Input: part model. Units: mm. Frame: model coordinates. A direction names the side the tool comes from. Coordinates: 2 decimals unless noted, no trailing zeros. Write each loop counter-clockwise with the first axis right and the second up, starting at its lowest first coordinate (ties: lowest second). Pieces come first, ordered by that corner, then holes. Notation, with made-up numbers: M 43,53 L 92,53 A23 cw 92,70 Z; hole C 21,-35.75 d1. An arc over 180 degrees is marked long. Write each question's results on one line, items separated by ' | '. Start each with the question number.
1. Section query B-B, the plane y = 27.5. Output: boundary loops of the cut face in (x, z), and give its area (3 significant figures).
2. Ray query, probe 1 along Z at (x, y) = (49, 41.5); probe 2 along Z at (x, y) = (61, 1); probe 3 along X at (y, z) = (34.5, 34.5). Return the intervals inside material, ascending.
3. Set-up query: faces 1 (the flat face through (66, 1, 21)), 2 (the flat face through (4, 2, 21)), 3 (the cylindrical face through (54.57, 0.6, 21.29)). Return all of +Z, -Z, +X, -X, +Y, -Y with unobstructed straight access to the full face (end or side cutting, diameter ignored); none if empty.
4. Section query C-C, the plane z = 21. Output: boundary loops of the cut face in (x, y), and give its area (3 significant figures).
5. First-contact query: pin 1 (6 mm diameter, centred on y = 21, z = 11.5, fed in from +X); pin 2 (4 mm diameter, centred on x = 5.5, z = 21, fed in from +Y); pin 3 (18 mm diameter, centred on y = 16.5, z = 23.5, fed in from -X). Flat tips, straight axial feed; report the tip coordinate or a pass-through.
6. Pull-direction query (X, two-part tool) for faces 4 (the flat face through (10, 22, 21)), 5 (the cylindrical face through (62.45, 0.99, 35.94)), 6 (the cylindrical face through (56.6, 2.57, 21.29)); classes: +X half, -X half, draft (parallel to the pull), parting line (faces both ways), or undercut.
7. Section query D-D, the plane x = 5. Output: boundary loops of the cut face in (y, z).
8. Section query A-A, the plane x = 33. Output: boundary loops of the cut face in (y, z).
```python
from build123d import *

# Parameters (mm, degrees)
BOSS_EXTRU_1_DEPTH      = 42
D_GAGEMENT_M2_51_D      = 2.9
D_GAGEMENT_M21_D        = 2.4
ENL_V_MAT_EXTRU_1_REACH = 90.792
ESQUISSE6_R             = 11
CONG_1_R                = 2


with BuildPart() as part:
    # Esquisse1 → Boss.-Extru.1 (new body)
    with BuildSketch(Plane.XY):
        Polygon((0, 0), (12, 0), (12, 40), (54, 40), (54, 0), (66, 0), (66, 2), (56, 2), (56, 42), (10, 42), (10, 2), (0, 2), align=None)
    extrude(amount=BOSS_EXTRU_1_DEPTH)

    # Dégagement M2.51 (through all)
    with Locations(Plane(origin=(0, 2, 0), x_dir=(1, 0, 0), z_dir=(0, 1, 0))):
        with Locations((5, -6), (5, -36), (61, -6), (61, -36)):
            Hole(D_GAGEMENT_M2_51_D / 2)

    # Dégagement M21 (through all)
    with Locations(Plane(origin=(0, 42, 0), x_dir=(1, 0, 0), z_dir=(0, 1, 0))):
        with Locations((17, -5), (49, -37), (17, -37), (49, -5)):
            Hole(D_GAGEMENT_M21_D / 2)

    # Esquisse6 → Enlèv. mat.-Extru.1 (cut, up to next)
    with BuildSketch(Plane(origin=(0, 42, 0), x_dir=(1, 0, 0), z_dir=(0, 1, 0)), mode=Mode.PRIVATE) as enl_v_mat_extru_1_sk1:
        with Locations(Location((33, -21, 0), (0, 0, 270))):
            Circle(ESQUISSE6_R)
    enl_v_mat_extru_1_tool1 = extrude(enl_v_mat_extru_1_sk1.sketch, amount=-ENL_V_MAT_EXTRU_1_REACH, mode=Mode.PRIVATE) & part.part
    add(enl_v_mat_extru_1_tool1.solids().sort_by_distance((33, 42, 21))[0], mode=Mode.SUBTRACT)

    # Congé1
    cong_1_edges = [part.edges().sort_by_distance(p)[0] for p in [
        (10, 2, 21),
        (10, 42, 21),
        (56, 42, 21),
        (56, 2, 21),
        (54, 0, 21),
        (12, 0, 21),
    ]]
    fillet(cong_1_edges, radius=CONG_1_R)


solid = part.part
```
Answer:
1) outline: M 10,0 L 12,0 L 12,42 L 10,42 Z; M 54,0 L 56,0 L 56,42 L 54,42 Z | area: 168 mm^2
2) probe 1: 0 to 3.8, 6.2 to 35.8, 38.2 to 42 | probe 2: 0 to 4.55, 7.45 to 34.55, 37.45 to 42 | probe 3: 10 to 12, 54 to 56
3) face 1: +Z, -Z, +X, +Y, -Y | face 2: +Z, -Z, -X, +Y | face 3: +Z, -Z, -Y
4) outline: M 0,0 L 10,0 A2 ccw 12,2 L 12,40 L 22,40 L 22,42 L 12,42 A2 ccw 10,40 L 10,4 A2 cw 8,2 L 0,2 Z; M 44,40 L 54,40 L 54,2 A2 ccw 56,0 L 66,0 L 66,2 L 58,2 A2 cw 56,4 L 56,40 A2 ccw 54,42 L 44,42 Z | area: 246 mm^2
5) pin 1: x = 56 | pin 2: y = 2 | pin 3: x = 10
6) face 4: -X half | face 5: undercut | face 6: +X half
7) outline: M 0,0 L 2,0 L 2,4.55 L 0,4.55 Z; M 0,7.45 L 2,7.45 L 2,34.55 L 0,34.55 Z; M 0,37.45 L 2,37.45 L 2,42 L 0,42 Z
8) outline: M 40,0 L 42,0 L 42,10 L 40,10 Z; M 40,32 L 42,32 L 42,42 L 40,42 Z
